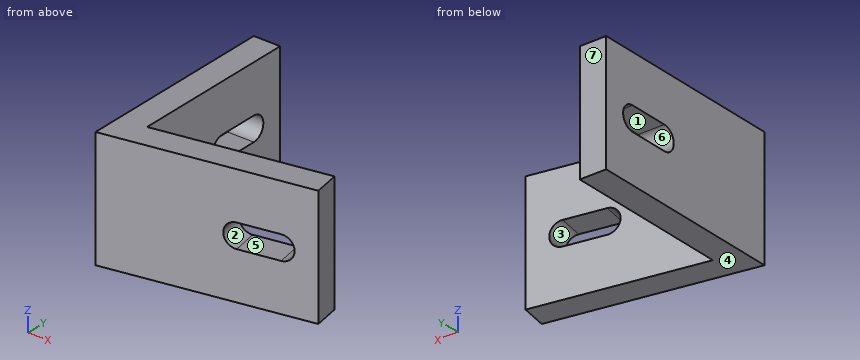
```python
from build123d import *

# Parameters (mm, degrees)
BOSS_EXTRUDE1_DEPTH      = 22.5
M8_CLEARANCE_SLOT1_DEPTH = 10


# Read off the part's stored shape, not the designer's step: M8 Clearance Slot1
with BuildPart() as part:
    # Sketch1 → Boss-Extrude1 (new, symmetric)
    with BuildSketch(Plane.XY):
        Polygon((0, 0), (73.860581476, 13.023613325), (72.124099699, 22.871690855), (10, 11.917535926), (10, 75), (0, 75), align=None)
    extrude(amount=BOSS_EXTRUDE1_DEPTH, both=True)

    # M8 Clearance Slot1 outline → M8 Clearance Slot1 (cut)
    with BuildSketch(Plane.YZ):
        with BuildLine():
            ThreePointArc((62.5, -4.5), (67, 0), (62.5, 4.5))
            Line((62.5, 4.5), (47.5, 4.5))
            ThreePointArc((47.5, 4.5), (43, 0), (47.5, -4.5))
            Line((47.5, -4.5), (62.5, -4.5))
        make_face()
    m8_clearance_slot1 = extrude(amount=M8_CLEARANCE_SLOT1_DEPTH, mode=Mode.SUBTRACT)

    # Mirror1: M8 Clearance Slot1 across plane
    add(m8_clearance_slot1.mirror(Plane(origin=(0, 0, 0), x_dir=(0, 0, 1), z_dir=(0.7660444431189772, -0.6427876096865405, 0))), mode=Mode.SUBTRACT)


solid = part.part
```
Read the model definition and answer for the solid it produces. Units are mm, in the model's axes. Face numbers are marked on the shaded views. A direction names the side the tool comes from. Coordinates: 2 decimals unless noted, no trailing zeros. Order: outer loops, then holes, each group sorted by start corner. A loop starts at its lowest first (then second) coordinate and runs counter-clockwise, first axis right, second up. Notation, with made-up numbers: (27, 67.25) - (76, 67.25) arc R18 ccw to (76, 100.25) - close; hole circle Ø8 at (-4, 57.5). An arc over 180 degrees is marked (long way). Answer as a JSON object with one key per item and string values. Group by question number.
Item 1: Section B-B (z = 0) is taken. Give the vertices of the cut face in (x, y).
Item 2: Section C-C (z = -12.5) is taken. Give the vertices of the cut face in (x, y), plus the area to 3 significant figures.
Item 3: The mould has two halves that part along Z. Classify the marked faces 4, 5, 6 and 7: +Z half, -Z half, draft (parallel to the pull), parting line (faces both ways), or undercut.
Item 4: Flat-ended cylindrical pins translate along their axes: P1, Ø10, axis at x = 66, z = 12, coming from the +Y side; P2, Ø10, axis at x = 19.5, z = 1, coming from the +Y side; P3, Ø12, axis at y = 16, z = -3, coming from the -X side; P4, Ø3, axis at x = 14, z = 12.5, coming from the -Y side. Find the tip coordinate at first contact, or state that the pin passes through.
Item 5: Consider probe 1 along X at (y, z) = (55.5, 11.5); probe 2 along Y at (x, z) = (69.5, 0.5); probe 3 along Y at (x, z) = (44, -19.5). Determine where each line is inside the solid, lowest interval first. Write a range as from..to.
Item 6: A tool of negligible diameter and unlimited length cuts with its end or side. For the marked faces 1, 2 and 3, from which of +Z, -Z, +X, -X, +Y, -Y can it reach the whole face along a straight path? Write none if from no direction.
Item 7: Section A-A (x = 54) is taken. Give the vertices of the cut face in (y, z), plus the area to 3 significant figures.
Item 8: Section D-D (x = 8) is taken. Give the vertices of the cut face in (y, z).
Results are:
{
 "1": {"outline": "(0, 0) - (42.35, 7.47) - (40.61, 17.31) - (10, 11.92) - (10, 43) - (0, 43) - close; (0, 67) - (10, 67) - (10, 75) - (0, 75) - close; (64.25, 21.48) - (65.98, 11.63) - (73.86, 13.02) - (72.12, 22.87) - close"},
 "2": {"outline": "(0, 0) - (73.86, 13.02) - (72.12, 22.87) - (10, 11.92) - (10, 75) - (0, 75) - close", "area": "1,380 mm^2"},
 "3": {"face 4": "-Z half", "face 5": "undercut", "face 6": "undercut", "face 7": "draft"},
 "4": {"P1": "stops at y = 22.67", "P2": "stops at y = 14.47", "P3": "stops at x = 0", "P4": "stops at y = 2.2"},
 "5": {"probe 1": "x = 0..10", "probe 2": "y = 12.25..22.41", "probe 3": "y = 7.76..17.91"},
 "6": {"face 1": "+X, -X", "face 2": "+Y", "face 3": "-Y"},
 "7": {"outline": "(9.52, -22.5) - (19.68, -22.5) - (19.68, -4.5) - (9.52, -4.5) - close; (9.52, 4.5) - (19.68, 4.5) - (19.68, 22.5) - (9.52, 22.5) - close", "area": "366 mm^2"},
 "8": {"outline": "(1.41, -22.5) - (75, -22.5) - (75, 22.5) - (1.41, 22.5) - close; hole (47.5, -4.5) - (62.5, -4.5) arc R4.5 ccw to (62.5, 4.5) - (47.5, 4.5) arc R4.5 ccw to start"}
}
